Geometry check sheet. Reference: the model listing, model coordinates, mm. Face numbers are marked on the shaded views. A direction names the side the tool comes from. Round coordinates to 2 decimals unless told otherwise and drop trailing zeros. Order: outer loops, then holes, each group sorted by start corner. A loop starts at its lowest first (then second) coordinate and runs counter-clockwise, first axis right, second up. Notation, with made-up numbers: (48, 4) - (101, 4) arc R26 ccw to (101, 40) - close; hole circle Ø6 at (60, 77). An arc over 180 degrees is marked (long way). Use a Markdown table: item, result. Add a question column.
(1) Section check C-C on x = 3.7. Give the number of separate pieces and of enclosed holes in the cut face, then the cut area to 3 significant figures.
(2) Section check B-B on y = 11. Record the boundary of the cut face in (x, z).
(3) Thickness scan on line 1 along X through (y, z) = (4, 8); line 2 along Z through (x, y) = (2.75, 0); line 3 along Z through (x, y) = (0.35, -5). Record the ranges inside material, lowest first. Write a range as [from, to].
(4) Section check D-D on z = 1. Record the boundary of the cut face in (x, y), then the cut area to 3 significant figures.
(5) Gauge pin test, flat ends, axial feed: P1, Ø12, axis at y = -13.5, z = -2.5, coming from the +X side; P2, Ø8, axis at y = -6, z = -10, coming from the -X side; P3, Ø1.5, axis at y = 5, z = 7, coming from the +X side. Record the tip position at first contact, or that the pin passes through.
(6) Section check A-A on z = 5. Record the boundary of the cut face in (x, y), then the cut area to 3 significant figures.
(7) Mould release check, pull along X, two halves, no side actions. Record for the marked faces 1, 2, 3 and 4: released by +X, released by -X, zero draft, split by the parting line, or undercut.
(8) Access from +Z, -Z, +X, -X, +Y, -Y to the whole of each face (thin tool, end or side, straight path). Record for the marked faces 5, 6, 7 and 8.
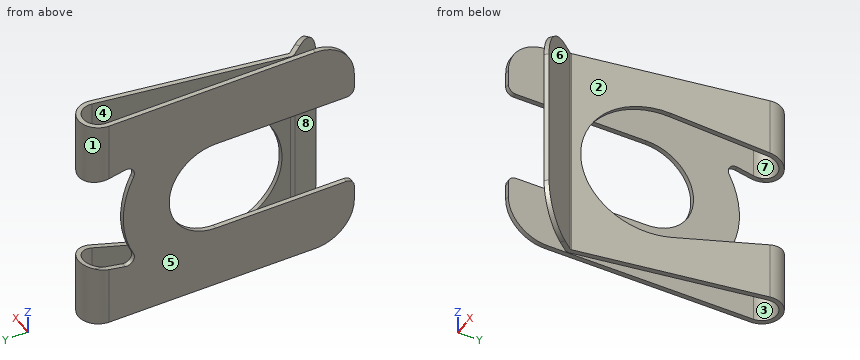
```python
from build123d import *

# Parameters (mm, degrees)
BOSS_EXTRUDE1_DEPTH      = 14
BOSS_EXTRUDE1_DEPTH_BACK = 14
CUT_EXTRUDE1_DEPTH       = 0.6
CUT_EXTRUDE2_DEPTH       = 5.4
CUT_EXTRUDE3_DEPTH       = 5.4
CUT_EXTRUDE4_DEPTH       = 0.6
CUT_EXTRUDE5_DEPTH       = 0.6
CUT_EXTRUDE6_DEPTH       = 0.6
CUT_EXTRUDE7_DEPTH       = 0.6
CUT_EXTRUDE8_DEPTH       = 1.2
CUT_EXTRUDE8_DEPTH_BACK  = 1.2


with BuildPart() as part:
    # Sketch1 → Boss-Extrude1 (new body, two sides)
    with BuildSketch(Plane.XY) as boss_extrude1_sk:
        with BuildLine():
            Line((0, 13.7), (0, -17.8))
            Line((0, -17.8), (0.6, -17.8))
            Line((0.6, -17.8), (0.6, 13.7))
            ThreePointArc((0.6, 13.7), (2.647893792, 15.594235314), (4.376976238, 13.405109849))
            Line((4.376976238, 13.405109849), (0.703859087, -9.974286111))
            ThreePointArc((0.703859087, -9.974286111), (0.724075997, -10.348603801), (0.895029628, -10.682216319))
            Line((0.895029628, -10.682216319), (5.036277977, -15.76853009))
            Line((5.036277977, -15.76853009), (5.501560288, -15.389699824))
            Line((5.501560288, -15.389699824), (1.360311939, -10.303386053))
            ThreePointArc((1.360311939, -10.303386053), (1.303327395, -10.19218188), (1.296588425, -10.067409316))
            Line((1.296588425, -10.067409316), (4.969705577, 13.311986643))
            ThreePointArc((4.969705577, 13.311986643), (2.694597095, 16.192414887), (0, 13.7))
        make_face()
    extrude(amount=BOSS_EXTRUDE1_DEPTH)
    extrude(boss_extrude1_sk.sketch, amount=-BOSS_EXTRUDE1_DEPTH_BACK)

    # Sketch2 → Cut-Extrude1 (cut)
    with BuildSketch(Plane(origin=(0, 0, 0), x_dir=(0, 0, -1), z_dir=(1, 0, 0))):
        with BuildLine():
            Line((-6, 0), (-6, -17.8))
            Line((-6, -17.8), (6, -17.8))
            Line((6, -17.8), (6, 0))
            ThreePointArc((6, 0), (0, 6), (-6, 0))
        make_face()
    extrude(amount=CUT_EXTRUDE1_DEPTH, mode=Mode.SUBTRACT)

    # Sketch3 → Cut-Extrude2 (cut)
    with BuildSketch(Plane(origin=(0.6, 0, 0), x_dir=(0, 0, -1), z_dir=(1, 0, 0))):
        with BuildLine():
            Line((8.832410113, 1.728736995), (6, 16.2))
            Line((6, 16.2), (-6, 16.2))
            Line((-6, 16.2), (-8.832410113, 1.728736995))
            ThreePointArc((-8.832410113, 1.728736995), (0, -9), (8.832410113, 1.728736995))
        make_face()
    extrude(amount=CUT_EXTRUDE2_DEPTH, mode=Mode.SUBTRACT)

    # Sketch4 → Cut-Extrude3 (cut)
    with BuildSketch(Plane(origin=(0.6, 0, 0), x_dir=(0, 0, -1), z_dir=(1, 0, 0))):
        with BuildLine():
            Line((6.88858316, 11.660078132), (6, 16.2))
            Line((6, 16.2), (-6, 16.2))
            Line((-6, 16.2), (-6.88858316, 11.660078132))
            ThreePointArc((-6.88858316, 11.660078132), (-6.507772079, 10.668422424), (-5.449281397, 10.579004313))
            ThreePointArc((-5.449281397, 10.579004313), (2.9e-08, 11.9), (5.449281448, 10.579004287))
            ThreePointArc((5.449281448, 10.579004287), (6.507772102, 10.668422441), (6.88858316, 11.660078132))
        make_face()
    extrude(amount=-CUT_EXTRUDE3_DEPTH, mode=Mode.SUBTRACT)

    # Sketch5 → Cut-Extrude4 (cut)
    with BuildSketch(Plane(origin=(0, 0, 0), x_dir=(0, 0, -1), z_dir=(1, 0, 0))):
        with BuildLine():
            Line((-14, -17.8), (-9, -17.8))
            ThreePointArc((-9, -17.8), (-12.535533906, -16.335533906), (-14, -12.8))
            Line((-14, -12.8), (-14, -17.8))
        make_face()
    extrude(amount=CUT_EXTRUDE4_DEPTH, mode=Mode.SUBTRACT)

    # Sketch6 → Cut-Extrude5 (cut)
    with BuildSketch(Plane(origin=(0, 0, 0), x_dir=(0, 0, -1), z_dir=(1, 0, 0))):
        with BuildLine():
            Line((9, -17.8), (14, -17.8))
            Line((14, -17.8), (14, -12.8))
            ThreePointArc((14, -12.8), (12.535533906, -16.335533906), (9, -17.8))
        make_face()
    extrude(amount=CUT_EXTRUDE5_DEPTH, mode=Mode.SUBTRACT)

    # Sketch7 → Cut-Extrude6 (cut)
    with BuildSketch(Plane(origin=(0, 0, 0), x_dir=(0, 0, -1), z_dir=(1, 0, 0))):
        with BuildLine():
            Line((6, -17.8), (7, -17.8))
            ThreePointArc((7, -17.8), (6.292893219, -17.507106781), (6, -16.8))
            Line((6, -16.8), (6, -17.8))
        make_face()
    extrude(amount=CUT_EXTRUDE6_DEPTH, mode=Mode.SUBTRACT)

    # Sketch8 → Cut-Extrude7 (cut)
    with BuildSketch(Plane(origin=(0, 0, 0), x_dir=(0, 0, -1), z_dir=(1, 0, 0))):
        with BuildLine():
            Line((-7, -17.8), (-6, -17.8))
            Line((-6, -17.8), (-6, -16.8))
            ThreePointArc((-6, -16.8), (-6.292893219, -17.507106781), (-7, -17.8))
        make_face()
    extrude(amount=CUT_EXTRUDE7_DEPTH, mode=Mode.SUBTRACT)

    # Sketch9 → Cut-Extrude8 (cut, two sides)
    with BuildSketch(Plane(origin=(-4.226709045, -3.441362969, 0), x_dir=(0, 0, -1), z_dir=(0.775470518, 0.631383778, 0))) as cut_extrude8_sk:
        with BuildLine():
            Line((-14, -10.380851015), (-19, -10.380851015))
            Line((-19, -10.380851015), (-19, -20.380851015))
            Line((-19, -20.380851015), (19, -20.380851015))
            Line((19, -20.380851015), (19, -10.380851015))
            Line((19, -10.380851015), (14, -10.380851015))
            ThreePointArc((14, -10.380851015), (12.535533906, -13.916384921), (9, -15.380851015))
            Line((9, -15.380851015), (-9, -15.380851015))
            ThreePointArc((-9, -15.380851015), (-12.535533906, -13.916384921), (-14, -10.380851015))
        make_face()
    extrude(amount=CUT_EXTRUDE8_DEPTH, mode=Mode.SUBTRACT)
    extrude(cut_extrude8_sk.sketch, amount=-CUT_EXTRUDE8_DEPTH_BACK, mode=Mode.SUBTRACT)


solid = part.part
```
Check sheet entries:
| question | item | result |
|---|---|---|
| 1 | separate pieces | 5 |
| 1 | enclosed holes | 0 |
| 1 | area | 84.8 mm2 |
| 2 | outline | (0, -14) - (0.6, -14) - (0.6, -6.79) - (0, -6.79) - close; (0, -4.54) - (0.6, -4.54) - (0.6, 4.54) - (0, 4.54) - close; (0, 6.79) - (0.6, 6.79) - (0.6, 14) - (0, 14) - close; (4, -14) - (4.61, -14) - (4.61, -7.02) - (4, -7.02) - close; (4, 7.02) - (4.61, 7.02) - (4.61, 14) - (4, 14) - close |
| 3 | line 1 | x = [0, 0.6] |
| 3 | line 2 | z = [-14, -9], [9, 14] |
| 3 | line 3 | z = [-14, -6], [6, 14] |
| 4 | outline | (0, 5.92) - (0.6, 5.92) - (0.6, 11.86) - (0, 11.86) - close; (0.7, -9.97) arc R0.9 ccw to (0.9, -10.68) - (5.02, -15.75) - (5.48, -15.37) - (1.36, -10.3) arc R0.3 cw to (1.3, -10.07) - (1.47, -8.94) - (0.87, -8.94) - close |
| 4 | area | 8.44 mm2 |
| 5 | P1 | stops at x = 5.48 |
| 5 | P2 | stops at x = 0 |
| 5 | P3 | stops at x = 0.6 |
| 6 | outline | (0, 3.32) - (0.6, 3.32) - (0.6, 10.8) - (0, 10.8) - close; (0.7, -9.97) arc R0.9 ccw to (0.9, -10.68) - (5.02, -15.75) - (5.48, -15.37) - (1.36, -10.3) arc R0.3 cw to (1.3, -10.07) - (1.7, -7.48) - (1.1, -7.48) - close |
| 6 | area | 10.3 mm2 |
| 7 | face 1 | split by the parting line |
| 7 | face 2 | released by +X |
| 7 | face 3 | undercut |
| 7 | face 4 | undercut |
| 8 | face 5 | +Z, -Z, -X, +Y, -Y |
| 8 | face 6 | +Z, -Z, +X |
| 8 | face 7 | +Z, -Z |
| 8 | face 8 | +Z, -Z, -Y |
